Could you check a few things on this model? Use its own coordinates, in mm. A direction names the side the tool comes from. Round coordinates to 2 decimals unless told otherwise and drop trailing zeros. Loops run counter-clockwise (first coordinate to the right, second up) from the corner with the lowest first, then second, coordinate; pieces in that order, holes last. Notation, with made-up numbers: (89.5, 84.25) -> (97.5, 84.25) arc R29 ccw to (97.5, 110.25) -> close; hole circle Ø8 at (51.25, -32). An arc over 180 degrees is marked (long way). One line per item, written item: value.
```python
from build123d import *

# Parameters (mm, degrees)
F0_W          = 12
F0_H          = 30
F0_R          = 1
F1_DEPTH      = 6
F2_R          = 12
F2_R_2        = 8.1
F3_DEPTH      = 42
F4_DEPTH      = 6.001
F5_W          = 12
F5_H          = 1.5
F6_DEPTH      = 24.001
F7_R          = 1.5
F8_DEPTH      = 15.001
F8_DEPTH_BACK = 15.001
F9_SIZE       = 1


with BuildPart() as f1:
    # F0 (on Top) → F1 (new body)
    with BuildSketch(Plane.XY):
        Rectangle(F0_W, F0_H)
        with Locations((-1.5, -12.5)):
            Circle(F0_R, mode=Mode.SUBTRACT)
        with Locations((-1.5, 12.5)):
            Circle(F0_R, mode=Mode.SUBTRACT)
    extrude(amount=F1_DEPTH)

    # F2 (on face) → F3 (join)
    with BuildSketch(Plane.XY.offset(6)):
        with Locations((6, 0)):
            Circle(F2_R)
        with Locations((6, 0)):
            Circle(F2_R_2, mode=Mode.SUBTRACT)
    extrude(amount=F3_DEPTH)

    # F4 (cut, through all): a face of the model
    f4_faces = [f1.faces().sort_by_distance(p)[0] for p in [
        (2.5622532292, 0, 6),
    ]]
    extrude(f4_faces, amount=-F4_DEPTH, mode=Mode.SUBTRACT)

    # F5 (on face) → F6 (cut, through all)
    with BuildSketch(Plane(origin=(-6, 0, 0), x_dir=(0, -1, 0), z_dir=(-1, 0, 0))):
        with Locations((0, 0.75)):
            Rectangle(F5_W, F5_H)
    extrude(amount=-F6_DEPTH, mode=Mode.SUBTRACT)

    # F7 (on Front) → F8 (cut, two sides)
    with BuildSketch(Plane.XZ) as f8_sk:
        with Locations((6, 32)):
            Circle(F7_R)
    extrude(amount=-F8_DEPTH, mode=Mode.SUBTRACT)
    extrude(f8_sk.sketch, amount=F8_DEPTH_BACK, mode=Mode.SUBTRACT)

    # F9
    f9_edges = [f1.edges().sort_by_distance(p)[0] for p in [
        (-6, 0, 48),
    ]]
    chamfer(f9_edges, length=F9_SIZE)


solid = f1.part
```
(1) On a 3-axis mill with a long thin cutter (end or side, diameter ignored), from which of +Z, -Z, +X, -X, +Y, -Y can I reach the whole of each face in a straight line? I mean faces 1 (the face through (-1, 11, 6)), 2 (the face through (6, 12, 3)), 3 (the face through (-3, 6, 1)). Say none if no direction works.
Results below:
face 1: +Z, -X, +Y
face 2: -Z, +X, +Y, -Y
face 3: -Z, +X, -X
(2) Imagine slicing it at C-C on z = 32. Write out the boundary of the cut face in (x, y), then the cut area to 3 significant figures.
Results below:
outline: (4.5, -11.91) -> (4.5, -7.96) arc R8.1 cw to (4.5, 7.96) -> (4.5, 11.91) arc R12 ccw to start; (7.5, -11.91) arc R12 ccw to (7.5, 11.91) -> (7.5, 7.96) arc R8.1 cw to (7.5, -7.96) -> close
area: 223 mm²
(3) We'd pull the mould along Z, two halves only. Please class faces 4 (the face through (0, -15, 3)), 5 (the face through (0, -10, 0)), 6 (the face through (5.675, -9.951, 30.536)): +Z half, -Z half, draft (parallel to the pull), parting line (faces both ways), or undercut.
Results below:
face 4: draft
face 5: -Z half
face 6: undercut
(4) Imagine slicing it at D-D on z = 10. Write out the boundary of the cut face in (x, y).
Results below:
outline: circle Ø24 at (6, 0); hole circle Ø16.2 at (6, 0)
(5) For pin 1 Ø4 at (x, y) = (-2.5, 5.5) entering from -Z; pin 2 Ø3 at (x, y) = (-1.5, 12.5) entering from +Z; pin 3 Ø4 at (y, z) = (-9.5, 25) entering from +X; pin 4 Ø5 at (y, z) = (-10, 2.5) entering from +X, each with a flat end and sliding along its axis, tell me the tip position at first contact or that it passes through.
Results below:
pin 1: stops at z = 0
pin 2: stops at z = 6
pin 3: stops at x = 15.37
pin 4: stops at x = 6
(6) Imagine slicing it at B-B on z = 5. Write out the boundary of the cut face in (x, y).
Results below:
outline: (-6, -15) -> (6, -15) -> (6, -8.1) arc R8.1 cw to (6, 8.1) -> (6, 15) -> (-6, 15) -> close; hole circle Ø2 at (-1.5, -12.5); hole circle Ø2 at (-1.5, 12.5)
(7) Please list where these lines run through material, in increasing order: L1, parallel to Y at x = 5.75, z = 10; L2, parallel to X at y = 0.25, z = 17.5; L3, parallel to Z at x = -3.5, y = -10.5.
Results below:
L1: y = -12 to -8.1, 8.1 to 12
L2: x = -6 to -2.1, 14.1 to 18
L3: z = 0 to 6
(8) Imagine slicing it at A-A on y = 12.5. Write out the boundary of the cut face in (x, z), then the cut area to 3 significant figures.
Results below:
outline: (-6, 0) -> (-2.5, 0) -> (-2.5, 6) -> (-6, 6) -> close; (-0.5, 0) -> (6, 0) -> (6, 6) -> (-0.5, 6) -> close
area: 60.0 mm²
